from build123d import *

# Parameters (mm, degrees)
SKETCH1_W           = 20
SKETCH1_H           = 20
BOSS_EXTRUDE1_DEPTH = 50
SKETCH3_W           = 20
SKETCH3_H           = 10
BOSS_EXTRUDE3_DEPTH = 20


with BuildPart() as part:
    # Sketch1 → Boss-Extrude1 (new body)
    with BuildSketch(Plane.XY):
        Rectangle(SKETCH1_W, SKETCH1_H)
    extrude(amount=BOSS_EXTRUDE1_DEPTH)

    # Sketch3 → Boss-Extrude3 (add)
    with BuildSketch(Plane(origin=(0, 10, 0), x_dir=(1, 0, 0), z_dir=(0, 1, 0))):
        with Locations((0, -5)):
            Rectangle(SKETCH3_W, SKETCH3_H)
    boss_extrude3 = extrude(amount=BOSS_EXTRUDE3_DEPTH)

    # Mirror2: Boss-Extrude3 across plane
    add(boss_extrude3.mirror(Plane.ZX))


solid = part.part
Verification items for the finished model (mm, model axes). A direction names the side the tool comes from. Coordinates: 2 decimals unless noted, no trailing zeros. Order: outer loops, then holes, each group sorted by start corner. A loop starts at its lowest first (then second) coordinate and runs counter-clockwise, first axis right, second up.
Item 1: Section check B-B, the plane z = 45. Enter the section's corners in (x, y).
Filled in:
outline: (-10, -10) - (10, -10) - (10, 10) - (-10, 10) - close
Item 2: Section check C-C, the plane y = 22. Enter the section's corners in (x, z).
Filled in:
outline: (-10, 0) - (10, 0) - (10, 10) - (-10, 10) - close
Item 3: Depth check by flat-ended pin: pin 1 (3 mm diameter, centred on x = -1.5, z = 17, fed in from +Y); pin 2 (8 mm diameter, centred on x = 2, z = 14.5, fed in from -Y); pin 3 (12 mm diameter, centred on x = 0, y = 8.5, fed in from -Z). Enter the tip coordinate at first touch or a pass-through.
Filled in:
pin 1: stops at y = 10
pin 2: stops at y = -10
pin 3: stops at z = 0
Item 4: Material ranges on L1, parallel to Y at x = -0.25, z = 25; L2, parallel to Z at x = -2.75, y = -15.5, recorded low to high.
Filled in:
L1: y = -10 to 10
L2: z = 0 to 10
Item 5: Section check A-A, the plane x = -4. Enter the section's corners in (y, z), then the cut area to 3 significant figures.
Filled in:
outline: (-30, 0) - (30, 0) - (30, 10) - (10, 10) - (10, 50) - (-10, 50) - (-10, 10) - (-30, 10) - close
area: 1,400 mm2
Item 6: Access from +Z, -Z, +X, -X, +Y, -Y to the whole of each face (thin tool, end or side, straight path). Record for faces 1 (the face through (-10, 0, 20)), 2 (the face through (0, -10, 30)), 3 (the face through (0, 10, 30)).
Filled in:
face 1: +Z, -Z, -X, +Y, -Y
face 2: +Z, +X, -X, -Y
face 3: +Z, +X, -X, +Y
